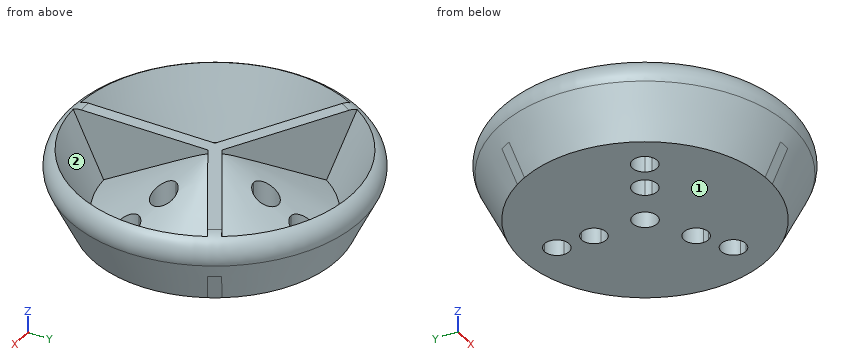
from build123d import *

# Parameters (mm, degrees)
F3_DEPTH = 6
F5_DEPTH = 6.0010001
F6_R     = 1
F7_DEPTH = 5


# Not quite as in the source:
# - a fillet or chamfer that OpenCascade refuses, or shapes differently, is made with other operations: its cross-section is extruded or revolved along the edge and cut away or added


with BuildPart() as f1:
    # F0 (on Front) → F1 (revolve)
    with BuildSketch(Plane.XZ):
        Polygon((0, 0), (10, 0), (8.7085954955, 0.7748427027), (0, 6), align=None)
        Polygon((8.7085954955, 0.7748427027), (10, 0), (12.905373238, 6), (11.2387675248, 6), align=None)
    revolve(axis=Axis((0, 0, 3), (0, 0, -1)))

    # F2 (on face) → F3 (join, through all)
    with BuildSketch(Plane.XY.offset(6)):
        with BuildLine():
            Line((0, -11.2387675248), (0, 0))
            Line((0, 0), (-9.7330581837, 5.6193837624))
            ThreePointArc((-9.7330581837, 5.6193837624), (-9.8556796151, 5.401432662), (-9.9734212913, 5.1808071981))
            Line((-9.9734212913, 5.1808071981), (-0.5, -0.2886751346))
            Line((-0.5, -0.2886751346), (-0.5, -11.2276397999))
            ThreePointArc((-0.5, -11.2276397999), (-0.2500619055, -11.2359852492), (0, -11.2387675248))
        make_face()
        with BuildLine():
            Line((9.7330581837, 5.6193837624), (0, 0))
            Line((0, 0), (0, -11.2387675248))
            ThreePointArc((0, -11.2387675248), (0.2500619055, -11.2359852492), (0.5, -11.2276397999))
            Line((0.5, -11.2276397999), (0.5, -0.2886751346))
            Line((0.5, -0.2886751346), (9.9734212913, 5.1808071981))
            ThreePointArc((9.9734212913, 5.1808071981), (9.8556796151, 5.401432662), (9.7330581837, 5.6193837624))
        make_face()
        with BuildLine():
            Line((-9.7330581837, 5.6193837624), (0, 0))
            Line((0, 0), (9.7330581837, 5.6193837624))
            ThreePointArc((9.7330581837, 5.6193837624), (9.6056177096, 5.8345525873), (9.4734212913, 6.0468326019))
            Line((9.4734212913, 6.0468326019), (0, 0.5773502692))
            Line((0, 0.5773502692), (-9.4734212913, 6.0468326019))
            ThreePointArc((-9.4734212913, 6.0468326019), (-9.6056177096, 5.8345525873), (-9.7330581837, 5.6193837624))
        make_face()
    extrude(amount=-F3_DEPTH)

    # F4 (on face) → F5 (cut, through all)
    with BuildSketch(Plane.XY.offset(6)):
        with BuildLine():
            ThreePointArc((7.1655671975, -3.5596918812), (6.4243862426, -2.5937660549), (5.2995417938, -3.0596918812))
            Line((5.2995417938, -3.0596918812), (7.0315926013, -4.0596918812))
            ThreePointArc((7.0315926013, -4.0596918812), (7.1314930238, -3.8185109263), (7.1655671975, -3.5596918812))
        make_face()
        with BuildLine():
            Line((7.0315926013, -4.0596918812), (5.2995417938, -3.0596918812))
            ThreePointArc((5.2995417938, -3.0596918812), (5.6655671975, -4.425717285), (7.0315926013, -4.0596918812))
        make_face()
        with BuildLine():
            ThreePointArc((4.5674909862, -2.0596918812), (3.8263100313, -1.0937660549), (2.7014655824, -1.5596918812))
            Line((2.7014655824, -1.5596918812), (4.43351639, -2.5596918812))
            ThreePointArc((4.43351639, -2.5596918812), (4.5334168125, -2.3185109263), (4.5674909862, -2.0596918812))
        make_face()
        with BuildLine():
            Line((4.43351639, -2.5596918812), (2.7014655824, -1.5596918812))
            ThreePointArc((2.7014655824, -1.5596918812), (3.0674909862, -2.925717285), (4.43351639, -2.5596918812))
        make_face()
        with BuildLine():
            ThreePointArc((-5.1655671975, -3.5596918812), (-5.1996413713, -3.3008728361), (-5.2995417938, -3.0596918812))
            Line((-5.2995417938, -3.0596918812), (-7.0315926013, -4.0596918812))
            ThreePointArc((-7.0315926013, -4.0596918812), (-5.9067481524, -4.5256177075), (-5.1655671975, -3.5596918812))
        make_face()
        with BuildLine():
            Line((-7.0315926013, -4.0596918812), (-5.2995417938, -3.0596918812))
            ThreePointArc((-5.2995417938, -3.0596918812), (-6.6655671975, -2.6936664774), (-7.0315926013, -4.0596918812))
        make_face()
        with BuildLine():
            ThreePointArc((-2.5674909862, -2.0596918812), (-2.6015651599, -1.8008728361), (-2.7014655824, -1.5596918812))
            Line((-2.7014655824, -1.5596918812), (-4.43351639, -2.5596918812))
            ThreePointArc((-4.43351639, -2.5596918812), (-3.3086719411, -3.0256177075), (-2.5674909862, -2.0596918812))
        make_face()
        with BuildLine():
            Line((-4.43351639, -2.5596918812), (-2.7014655824, -1.5596918812))
            ThreePointArc((-2.7014655824, -1.5596918812), (-4.0674909862, -1.1936664774), (-4.43351639, -2.5596918812))
        make_face()
        with BuildLine():
            ThreePointArc((0, 8.1193837624), (-1, 7.1193837624), (0, 6.1193837624))
            Line((0, 6.1193837624), (0, 8.1193837624))
        make_face()
        with BuildLine():
            Line((0, 8.1193837624), (0, 6.1193837624))
            ThreePointArc((0, 6.1193837624), (0.7071067812, 6.4122769812), (1, 7.1193837624))
            ThreePointArc((1, 7.1193837624), (0.7071067812, 7.8264905436), (0, 8.1193837624))
        make_face()
        with BuildLine():
            ThreePointArc((0, 5.1193837624), (-1, 4.1193837624), (0, 3.1193837624))
            Line((0, 3.1193837624), (0, 5.1193837624))
        make_face()
        with BuildLine():
            Line((0, 5.1193837624), (0, 3.1193837624))
            ThreePointArc((0, 3.1193837624), (0.7071067812, 3.4122769812), (1, 4.1193837624))
            ThreePointArc((1, 4.1193837624), (0.7071067812, 4.8264905436), (0, 5.1193837624))
        make_face()
    extrude(amount=-F5_DEPTH, mode=Mode.SUBTRACT)

    # F6 (on face) → F7 (cut)
    with BuildSketch(Plane(origin=(0, 0, 0), x_dir=(1, 0, 0), z_dir=(0, 0, -1))):
        Circle(F6_R)
    extrude(amount=-F7_DEPTH, mode=Mode.SUBTRACT)

    # F8: fillet of radius 1.5 on 1 edges, made by hand

    # F8_s1 → F8_t2 (revolve, cut)
    with BuildSketch(Plane.XZ):
        with BuildLine():
            ThreePointArc((11.8624735894, 3.8462671131), (11.7833686143, 5.2966808237), (10.5124242153, 6))
            Line((10.5124242153, 6), (12.905373238, 6))
            Line((12.905373238, 6), (11.8624735894, 3.8462671131))
        make_face()
    revolve(axis=Axis((0, 0, 6), (0, 0, -1)), mode=Mode.SUBTRACT)

    # F0 (on Front) → F9 (revolve, cut)
    with BuildSketch(Plane.XZ):
        Polygon((12.905373238, 6), (10, 0), (13.7833622578, 0), (16.6887354958, 6), align=None)
    revolve(axis=Axis((0, 0, 3), (0, 0, -1)), mode=Mode.SUBTRACT)


solid = f1.part
Input: part model. Units: mm. Frame: model coordinates. Face numbers are marked on the shaded views. Round coordinates to 2 decimals unless told otherwise and drop trailing zeros.
1) Draft query along Y for the marked faces 1 and 2. Return one class per face: pulls with the +Y half, pulls with the -Y half, needs draft (parallel to the pull), parting line crosses it, or undercut.
2) Ray query, L1, parallel to Y at x = 4.75, z = 1.75; L2, parallel to X at y = 0, z = 2.1; L3, parallel to Y at x = -6.25, z = 5.5. Return the intervals inside material, ascending.
3) Contact query for flat-ended pins moving along their axis: P1, Ø4, axis at x = 6, y = 1, coming from the -Z side; P2, Ø5, axis at x = -1.5, y = 5.5, coming from the +Z side; P3, Ø1.6, axis at y = -6.5, z = 4.5, coming from the -X side. Output: stop coordinate, or through.
Geometry says:
1. face 1: needs draft
1. face 2: undercut
2. L1: y = -9.75 to -7.86, -5.25 to 5.25, 7.86 to 9.75
2. L2: x = -11.02 to -9.35, -6.5 to -1, 1 to 6.5, 9.35 to 11.02
2. L3: y = -9.81 to -9.05, 3.03 to 4.19, 9.05 to 9.81
3. P1: stops at z = 0
3. P2: stops at z = 4.08
3. P3: stops at x = -10.57
